Part print with two shaded views. Sizes in mm from the minimum x, y, z corner. Round coordinates to 2 decimals unless told otherwise and drop trailing zeros. Order: outer loops, then holes, each group sorted by start corner. A loop starts at its lowest first (then second) coordinate and runs counter-clockwise, first axis right, second up. Notation, with made-up numbers: (89.5, -9) -> (130.5, -9) arc R24 cw to (130.5, 23) -> close; hole circle Ø11 at (50.5, -30). An arc over 180 degrees is marked (long way). Use a Markdown table: item, result. Add a question column.
Item 1: Two-plate mould, pull along Y, no slides. Class the marked faces 1, 2 and 3: released by +Y, released by -Y, zero draft, split by the parting line, or undercut.
Item 2: Slice it at A-A, the plane y = 8. Give the cut face in (x, z).
Item 3: Slice it at D-D, the plane z = 5.75. Give the cut face in (x, y), plus the area to 3 significant figures.
Item 4: Slice it at B-B, the plane y = 16. Give the cut face in (x, z).
Item 5: Pin check, flat tips, straight feed: pin 1 (3 mm diameter, centred on x = 6, y = 10, fed in from -Z); pin 2 (0.6 mm diameter, centred on x = 13.5, z = 0.5, fed in from -Y); pin 3 (0.6 mm diameter, centred on y = 18, z = 1, fed in from +X). Stop position of each tip, or through.
Item 6: Probe L1, parallel to X at y = 8, z = 4.05; L2, parallel to Z at x = 6.5, y = 27.5; L3, parallel to Y at x = 13.5, z = 4.25. List the from-to ranges inside material, lowest first.
Item 7: Slice it at C-C, the plane x = 12.75. Give the cut face in (y, z), plus the area to 4 significant figures.
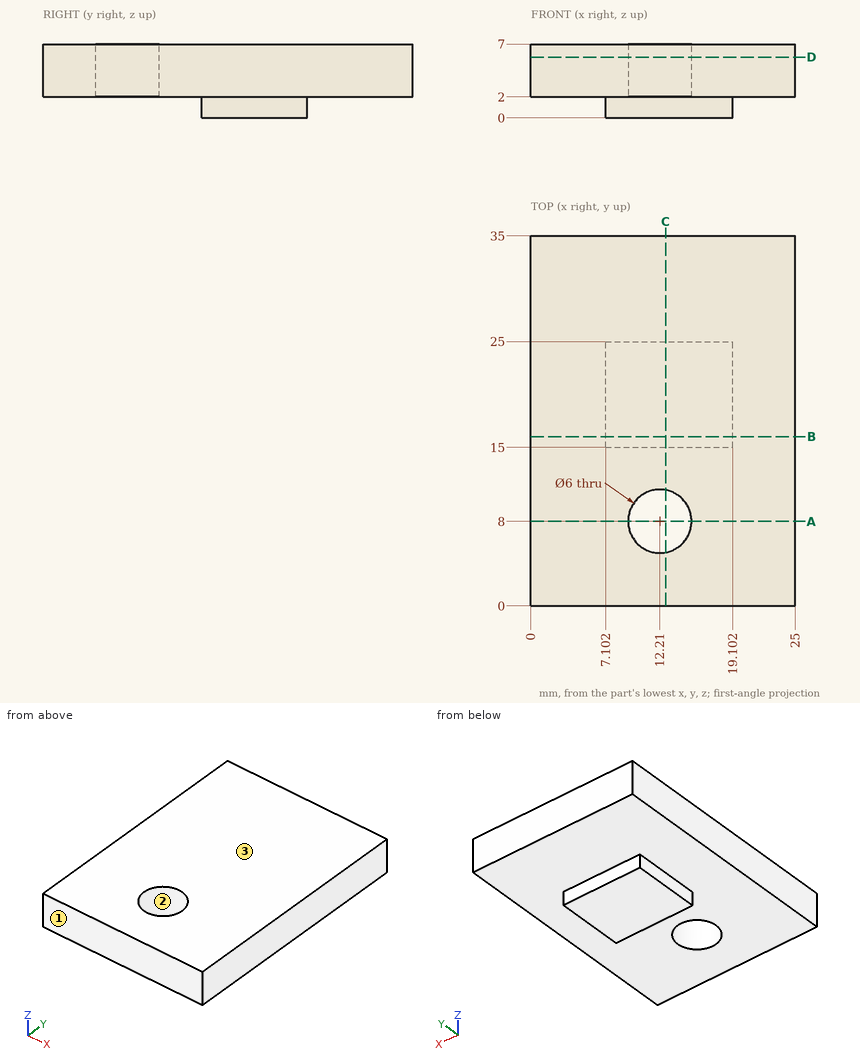
Check sheet entries:
| question | item | result |
|---|---|---|
| 1 | face 1 | released by -Y |
| 1 | face 2 | undercut |
| 1 | face 3 | zero draft |
| 2 | outline | (0, 2) -> (9.21, 2) -> (9.21, 7) -> (0, 7) -> close; (15.21, 2) -> (25, 2) -> (25, 7) -> (15.21, 7) -> close |
| 3 | outline | (0, 0) -> (25, 0) -> (25, 35) -> (0, 35) -> close; hole circle Ø6 at (12.21, 8) |
| 3 | area | 847 mm2 |
| 4 | outline | (0, 2) -> (7.1, 2) -> (7.1, 0) -> (19.1, 0) -> (19.1, 2) -> (25, 2) -> (25, 7) -> (0, 7) -> close |
| 5 | pin 1 | z = 2 |
| 5 | pin 2 | y = 15 |
| 5 | pin 3 | x = 19.1 |
| 6 | L1 | 0 to 9.21, 15.21 to 25 |
| 6 | L2 | 2 to 7 |
| 6 | L3 | 0 to 5.29, 10.71 to 35 |
| 7 | outline | (0, 2) -> (5.05, 2) -> (5.05, 7) -> (0, 7) -> close; (10.95, 2) -> (15, 2) -> (15, 0) -> (25, 0) -> (25, 2) -> (35, 2) -> (35, 7) -> (10.95, 7) -> close |
| 7 | area | 165.5 mm2 |
